Check sheet for the modelled part. Datum: model origin and axes. Units: mm. A direction names the side the tool comes from. Round coordinates to 2 decimals unless told otherwise and drop trailing zeros. Write item = value, one per line.
from build123d import *
from build123d.topology import SkipClean

# Parameters (mm, degrees)
SKETCH_1_W                = 40
SKETCH_1_H                = 40
SKETCH_1_R                = 1.55
EXTRUDE_2_DEPTH           = 3
CUT_EXTRUDE_1_DEPTH       = 1.5
SKETCH_2_W                = 3
SKETCH_2_H                = 3
EXTRUDE_7_DEPTH           = 45
SKETCH_5_W                = 40
SKETCH_5_H                = 3
EXTRUDE_8_DEPTH           = 40
SKETCH_6_R                = 12.5
CUT_EXTRUDE_2_DEPTH       = 4
CUT_EXTRUDE_START         = -4
CUT_EXTRUDE_3_DEPTH       = 4
SKETCH_8_R                = 5
CUT_EXTRUDE_4_DEPTH       = 4
SKETCH_9_R                = 2.5
CUT_EXTRUDE_5_DEPTH       = 4
SKETCH_10_W               = 1.5
SKETCH_10_H               = 34
SKETCH_10_W_2             = 34
SKETCH_10_H_2             = 1.5
EXTRUDE_10_DEPTH          = 45
CUT_EXTRUDE_12_DEPTH      = 63.507999
CUT_EXTRUDE_12_DEPTH_BACK = 4
CUT_EXTRUDE_13_DEPTH      = 4
CUT_EXTRUDE_13_DEPTH_BACK = 64.442888
CUT_EXTRUDE_15_DEPTH      = 10
CUT_EXTRUDE_15_DEPTH_BACK = 64.442888
SKETCH_24_5_R             = 1.85
SKETCH_24_5_R_2           = 5.5
CUT_EXTRUDE_16_DEPTH      = 10
CUT_EXTRUDE_16_DEPTH_BACK = 64.442888
SKETCH_25_R               = 5.5
SKETCH_25_R_2             = 1.85
SKETCH_27_W               = 60
SKETCH_27_H               = 60
SKETCH_27_R               = 1.6
EXTRUDE_13_DEPTH          = 3
FILLET_1_R                = 2
FILLET_2_R                = 5
SKETCH_28_R               = 13
CUT_EXTRUDE_17_DEPTH      = 10


with BuildPart() as part:
    # Sketch 1 → Extrude 2 (new body)
    with BuildSketch(Plane(origin=(0, 0, 0), x_dir=(1, 0, 0), z_dir=(0, 1, 0))):
        Rectangle(SKETCH_1_W, SKETCH_1_H)
        with Locations(Location((0, 8.5, 0), (0, 0, 270))):
            Circle(SKETCH_1_R, mode=Mode.SUBTRACT)
        with Locations(Location((8.5, 0, 0), (0, 0, 270))):
            Circle(SKETCH_1_R, mode=Mode.SUBTRACT)
        with Locations(Location((0, -8.5, 0), (0, 0, 270))):
            Circle(SKETCH_1_R, mode=Mode.SUBTRACT)
        with Locations(Location((-8.5, 0, 0), (0, 0, 270))):
            Circle(SKETCH_1_R, mode=Mode.SUBTRACT)
    extrude(amount=-EXTRUDE_2_DEPTH)

    # Sketch 1_6 → Cut-Extrude 1 (cut)
    with BuildSketch(Plane(origin=(0, 0, 0), x_dir=(1, 0, 0), z_dir=(0, 1, 0))):
        with BuildLine():
            ThreePointArc((4, 0), (2.828427, 2.828427), (0, 4))
            Line((0, 4), (0, -4))
            ThreePointArc((0, -4), (2.828427, -2.828427), (4, 0))
        make_face()
        with BuildLine():
            Line((0, -4), (0, 4))
            ThreePointArc((0, 4), (-4, 0), (0, -4))
        make_face()
    extrude(amount=-CUT_EXTRUDE_1_DEPTH, mode=Mode.SUBTRACT)

    # Sketch 2 → Extrude 7 (add)
    with BuildSketch(Plane(origin=(0, 0, 0), x_dir=(1, 0, 0), z_dir=(0, 1, 0))):
        with Locations((-18.5, 18.5)):
            Rectangle(SKETCH_2_W, SKETCH_2_H)
        with Locations((18.5, 18.5)):
            Rectangle(SKETCH_2_W, SKETCH_2_H)
        with Locations((18.5, -18.5)):
            Rectangle(SKETCH_2_W, SKETCH_2_H)
        with Locations((-18.5, -18.5)):
            Rectangle(SKETCH_2_W, SKETCH_2_H)
    extrude(amount=EXTRUDE_7_DEPTH)

    # Sketch 5 → Extrude 8 (add)
    with BuildSketch(Plane.ZY.offset(20)):
        with Locations((0, 43.5)):
            Rectangle(SKETCH_5_W, SKETCH_5_H)
    extrude(amount=-EXTRUDE_8_DEPTH)

    # Sketch 6 → Cut-Extrude 2 (cut)
    with BuildSketch(Plane(origin=(0, 45, 0), x_dir=(1, 0, 0), z_dir=(0, 1, 0))):
        with Locations(Location((0, 0, 0), (0, 0, 270))):
            Circle(SKETCH_6_R)
    extrude(amount=-CUT_EXTRUDE_2_DEPTH, mode=Mode.SUBTRACT)

    # Sketch 7 → Cut-Extrude 3 (cut)
    with SkipClean():  # the faces are left unmerged after this step: merging them gives an invalid solid
        with BuildSketch(Plane.XZ.offset(3).offset(CUT_EXTRUDE_START)):
            with BuildLine():
                ThreePointArc((-4, 0), (-2.828427, -2.828427), (0, -4))
                Line((0, -4), (0, 0))
                Line((0, 0), (-4, 0))
            make_face()
            with BuildLine():
                Line((0, 0), (0, -4))
                ThreePointArc((0, -4), (2.828427, -2.828427), (4, 0))
                ThreePointArc((4, 0), (0, 4), (-4, 0))
                Line((-4, 0), (0, 0))
            make_face()
        extrude(amount=CUT_EXTRUDE_3_DEPTH, mode=Mode.SUBTRACT)

    # Sketch 8 → Cut-Extrude 4 (cut)
    with SkipClean():  # the faces are left unmerged after this step: merging them gives an invalid solid
        with BuildSketch(Plane.XZ.offset(3)):
            with Locations(Location((-12, 12, 0), (0, 0, 270))):
                Circle(SKETCH_8_R)
            with Locations(Location((12, 12, 0), (0, 0, 270))):
                Circle(SKETCH_8_R)
            with Locations(Location((12, -12, 0), (0, 0, 270))):
                Circle(SKETCH_8_R)
            with Locations(Location((-12, -12, 0), (0, 0, 270))):
                Circle(SKETCH_8_R)
        extrude(amount=-CUT_EXTRUDE_4_DEPTH, mode=Mode.SUBTRACT)

    # Sketch 9 → Cut-Extrude 5 (cut)
    with SkipClean():  # the faces are left unmerged after this step: merging them gives an invalid solid
        with BuildSketch(Plane(origin=(0, 45, 0), x_dir=(1, 0, 0), z_dir=(0, 1, 0))):
            with Locations(Location((-12.727922, 12.727922, 0), (0, 0, 270))):
                Circle(SKETCH_9_R)
            with Locations(Location((12.727922, 12.727922, 0), (0, 0, 270))):
                Circle(SKETCH_9_R)
            with Locations(Location((12.727922, -12.727922, 0), (0, 0, 270))):
                Circle(SKETCH_9_R)
            with Locations(Location((-12.727922, -12.727922, 0), (0, 0, 270))):
                Circle(SKETCH_9_R)
        extrude(amount=-CUT_EXTRUDE_5_DEPTH, mode=Mode.SUBTRACT)

    # Sketch 10 → Extrude 10 (add)
    with SkipClean():  # the faces are left unmerged after this step: merging them gives an invalid solid
        with BuildSketch(Plane(origin=(0, 0, 0), x_dir=(1, 0, 0), z_dir=(0, 1, 0))):
            with Locations((19.25, 0)):
                Rectangle(SKETCH_10_W, SKETCH_10_H)
            with Locations((0, -19.25)):
                Rectangle(SKETCH_10_W_2, SKETCH_10_H_2)
            with Locations((-19.25, 0)):
                Rectangle(SKETCH_10_W, SKETCH_10_H)
            with Locations((0, 19.25)):
                Rectangle(SKETCH_10_W_2, SKETCH_10_H_2)
        extrude(amount=EXTRUDE_10_DEPTH)

    # Sketch 20 → Cut-Extrude 12 (cut, two sides: drawn at the far end of the back side and taken through both)
    with SkipClean():  # the faces are left unmerged after this step: merging them gives an invalid solid
        with BuildSketch(Plane(origin=(0, 0, 18.5), x_dir=(-1, 0, 0), z_dir=(0, 0, -1)).offset(-CUT_EXTRUDE_12_DEPTH_BACK)):
            with BuildLine():
                Line((-2.45, 36.5), (-2.45, 5.5))
                ThreePointArc((-2.45, 5.5), (0, 3.05), (2.45, 5.5))
                Line((2.45, 5.5), (2.45, 36.5))
                ThreePointArc((2.45, 36.5), (0, 38.95), (-2.45, 36.5))
            make_face()
        extrude(amount=CUT_EXTRUDE_12_DEPTH + CUT_EXTRUDE_12_DEPTH_BACK, mode=Mode.SUBTRACT)

    # Sketch 24 → Cut-Extrude 13 (cut, two sides: drawn at the far end of the back side and taken through both)
    with SkipClean():  # the faces are left unmerged after this step: merging them gives an invalid solid
        with BuildSketch(Plane(origin=(20, 0, 0), x_dir=(0, 0, -1), z_dir=(1, 0, 0)).offset(-CUT_EXTRUDE_13_DEPTH_BACK)):
            with BuildLine():
                Line((-2.45, 36.5), (-2.45, 5.5))
                ThreePointArc((-2.45, 5.5), (0, 3.05), (2.45, 5.5))
                Line((2.45, 5.5), (2.45, 36.5))
                ThreePointArc((2.45, 36.5), (0, 38.95), (-2.45, 36.5))
            make_face()
        extrude(amount=CUT_EXTRUDE_13_DEPTH + CUT_EXTRUDE_13_DEPTH_BACK, mode=Mode.SUBTRACT)

    # Sketch 24_5 → Cut-Extrude 15 (cut, two sides: drawn at the far end of the back side and taken through both)
    with SkipClean():  # the faces are left unmerged after this step: merging them gives an invalid solid
        with BuildSketch(Plane(origin=(20, 0, 0), x_dir=(0, 0, -1), z_dir=(1, 0, 0)).offset(-CUT_EXTRUDE_15_DEPTH_BACK)):
            with Locations((-11.45, 35)):
                Circle(SKETCH_24_5_R)
            with Locations(Location((-11.45, 7, 0), (0, 0, 180))):
                Circle(SKETCH_24_5_R)
            with Locations((11.45, 7)):
                Circle(SKETCH_24_5_R)
            with Locations(Location((11.45, 35, 0), (0, 0, 180))):
                Circle(SKETCH_24_5_R)
            with Locations((-11.35, 21)):
                Circle(SKETCH_24_5_R_2)
            with Locations(Location((11.35, 21, 0), (0, 0, 180))):
                Circle(SKETCH_24_5_R_2)
        extrude(amount=CUT_EXTRUDE_15_DEPTH + CUT_EXTRUDE_15_DEPTH_BACK, mode=Mode.SUBTRACT)

    # Sketch 25 → Cut-Extrude 16 (cut, two sides: drawn at the far end of the back side and taken through both)
    with SkipClean():  # the faces are left unmerged after this step: merging them gives an invalid solid
        with BuildSketch(Plane(origin=(0, 0, -20), x_dir=(-1, 0, 0), z_dir=(0, 0, -1)).offset(-CUT_EXTRUDE_16_DEPTH_BACK)):
            with Locations((-11.45, 21)):
                Circle(SKETCH_25_R)
            with Locations((11.45, 21)):
                Circle(SKETCH_25_R)
            with Locations((-11.45, 35)):
                Circle(SKETCH_25_R_2)
            with Locations((-11.45, 7)):
                Circle(SKETCH_25_R_2)
            with Locations((11.45, 7)):
                Circle(SKETCH_25_R_2)
            with Locations((11.45, 35)):
                Circle(SKETCH_25_R_2)
        extrude(amount=CUT_EXTRUDE_16_DEPTH + CUT_EXTRUDE_16_DEPTH_BACK, mode=Mode.SUBTRACT)

    # Sketch 27 → Extrude 13 (add)
    with BuildSketch(Plane.XZ.offset(3)):
        Rectangle(SKETCH_27_W, SKETCH_27_H)
        with Locations(Location((-15, -25, 0), (0, 0, 270))):
            Circle(SKETCH_27_R, mode=Mode.SUBTRACT)
        with Locations(Location((15, -25, 0), (0, 0, 270))):
            Circle(SKETCH_27_R, mode=Mode.SUBTRACT)
        with Locations(Location((25, -25, 0), (0, 0, 270))):
            Circle(SKETCH_27_R, mode=Mode.SUBTRACT)
        with Locations(Location((25, 25, 0), (0, 0, 270))):
            Circle(SKETCH_27_R, mode=Mode.SUBTRACT)
        with Locations(Location((15, 25, 0), (0, 0, 270))):
            Circle(SKETCH_27_R, mode=Mode.SUBTRACT)
        with Locations(Location((-15, 25, 0), (0, 0, 270))):
            Circle(SKETCH_27_R, mode=Mode.SUBTRACT)
        with Locations(Location((-25, 25, 0), (0, 0, 270))):
            Circle(SKETCH_27_R, mode=Mode.SUBTRACT)
        with Locations(Location((-25, -25, 0), (0, 0, 270))):
            Circle(SKETCH_27_R, mode=Mode.SUBTRACT)
        Polygon((-10, 20), (20, 20), (20, -20), (-20, -20), (-20, 20), align=None, mode=Mode.SUBTRACT)
    extrude(amount=-EXTRUDE_13_DEPTH)

    # Fillet 1
    fillet_1_edges = [part.edges().sort_by_distance(p)[0] for p in [
        (-20, 0, 0),
        (0, 0, -20),
        (20, 0, 0),
        (0, 0, 20),
    ]]
    fillet(fillet_1_edges, radius=FILLET_1_R)

    # Fillet 2
    fillet_2_edges = [part.edges().sort_by_distance(p)[0] for p in [
        (30, -1.5, -30),
        (-30, -1.5, -30),
        (-30, -1.5, 30),
        (30, -1.5, 30),
    ]]
    fillet(fillet_2_edges, radius=FILLET_2_R)

    # Sketch 28 → Cut-Extrude 17 (cut)
    with SkipClean():  # the faces are left unmerged after this step: merging them gives an invalid solid
        with BuildSketch(Plane(origin=(0, 45, 0), x_dir=(1, 0, 0), z_dir=(0, 1, 0))):
            with Locations(Location((0, 0, 0), (0, 0, 270))):
                Circle(SKETCH_28_R)
        extrude(amount=-CUT_EXTRUDE_17_DEPTH, mode=Mode.SUBTRACT)


solid = part.part
(1) Release check for a two-part mould opening along Z. For faces 5 (the flat face through (2.45, 21, -19)), 6 (the flat face through (-5, 24, 20)), 7 (the flat face through (-4, 21, 18.5)) record: pulls with the +Z half, pulls with the -Z half, needs draft (parallel to the pull), parting line crosses it, or undercut.
Worked answers:
face_5 = needs draft
face_6 = pulls with the +Z half
face_7 = undercut
(2) Material ranges on L1, parallel to Y at x = -19.45, z = -11.45; L2, parallel to X at y = -1.25, z = 0; L3, parallel to X at y = -1, z = -25, recorded low to high. Write a range as [from, to].
Worked answers:
L1 = [-3, 5.15], [8.85, 15.5], [26.5, 33.15], [36.85, 45]
L2 = [-30, -10.05], [-6.95, -4], [4, 6.95], [10.05, 30]
L3 = [-30, -26.6], [-23.4, -16.6], [-13.4, 13.4], [16.6, 23.4], [26.6, 30]
(3) Go/stop test with flat-tipped pins: P1, Ø4, axis at y = 11, z = 7.5, coming from the +X side; P2, Ø8, axis at y = 23.5, z = 17.5, coming from the -X side; P3, Ø12, axis at x = 17.5, y = 24.5, coming from the -Z side. Record where each tip stops, or that it passes through.
Worked answers:
P1 = 20
P2 = -20
P3 = -20
(4) Sectioned sample at A-A on y = 12.5. Count the separate pieces of the cut face and the enclosed holes in it, then the cut area to 3 significant figures.
Worked answers:
separate_pieces = 4
enclosed_holes = 0
area = 211 mm²
(5) Access from +Z, -Z, +X, -X, +Y, -Y to the whole of each face (thin tool, end or side, straight path). Record for faces 1 (the cylindrical face through (0.05, 3.05, -19.24)), 2 (the flat face through (-18, 21, -17)), 3 (the cylindrical face through (-10.5, -1.52, -16.77)), 4 (the cylindrical face through (19.24, 38.95, -0.05)).
Worked answers:
face_1 = +Z, -Z
face_2 = none
face_3 = -Y
face_4 = +X, -X
